from build123d import *

# Parameters (mm, degrees)
BOSS_EXTRUDE1_DEPTH     = 30
CUT_EXTRUDE1_DEPTH      = 72.944422994
CUT_EXTRUDE1_DEPTH_BACK = 4
SKETCH2_R               = 5
SKETCH3_R               = 2.25
CUT_EXTRUDE2_DEPTH      = 74.484692406
CHAMFER1_SIZE           = 1.5
SKETCH4_R               = 1.355
CUT_EXTRUDE3_DEPTH      = 10


with BuildPart() as part:
    # Sketch1 → Boss-Extrude1 (new body)
    with BuildSketch(Plane.XY):
        with BuildLine():
            Line((-35, -12), (-35, 12))
            ThreePointArc((-35, 12), (-34.414213562, 13.414213562), (-33, 14))
            Line((-33, 14), (33, 14))
            ThreePointArc((33, 14), (34.414213562, 13.414213562), (35, 12))
            Line((35, 12), (35, -12))
            ThreePointArc((35, -12), (35.585786438, -13.414213562), (37, -14))
            Line((37, -14), (45, -14))
            Line((45, -14), (45, 8))
            ThreePointArc((45, 8), (46.171572875, 10.828427125), (49, 12))
            Line((49, 12), (56, 12))
            ThreePointArc((56, 12), (58.828427125, 13.171572875), (60, 16))
            Line((60, 16), (60, 24))
            Line((60, 24), (33, 24))
            Line((33, 24), (-33, 24))
            Line((-33, 24), (-60, 24))
            Line((-60, 24), (-60, 16))
            ThreePointArc((-60, 16), (-58.828427125, 13.171572875), (-56, 12))
            Line((-56, 12), (-49, 12))
            ThreePointArc((-49, 12), (-46.171572875, 10.828427125), (-45, 8))
            Line((-45, 8), (-45, -14))
            Line((-45, -14), (-37, -14))
            ThreePointArc((-37, -14), (-35.585786438, -13.414213562), (-35, -12))
        make_face()
    extrude(amount=BOSS_EXTRUDE1_DEPTH)

    # Sketch2 → Cut-Extrude1 (cut, two sides: drawn at the far end of the back side and taken through both)
    with BuildSketch(Plane.XZ.offset(-12).offset(-CUT_EXTRUDE1_DEPTH_BACK)):
        with Locations(Location((-52.5, 15, 0), (0, 0, 134.427004004))):
            Circle(SKETCH2_R)
        with Locations(Location((52.5, 15, 0), (0, 0, 225.572995999))):
            Circle(SKETCH2_R)
    extrude(amount=CUT_EXTRUDE1_DEPTH + CUT_EXTRUDE1_DEPTH_BACK, mode=Mode.SUBTRACT)

    # Sketch3 → Cut-Extrude2 (cut, through all)
    with BuildSketch(Plane.XZ.offset(-16)):
        with Locations((-52.5, 15)):
            Circle(SKETCH3_R)
        with Locations((52.5, 15)):
            Circle(SKETCH3_R)
    extrude(amount=-CUT_EXTRUDE2_DEPTH, mode=Mode.SUBTRACT)

    # Chamfer1
    chamfer1_edges = [part.edges().sort_by_distance(p)[0] for p in [
        (-54.75, 16, 15),
        (50.25, 16, 15),
    ]]
    chamfer(chamfer1_edges, length=CHAMFER1_SIZE)

    # Sketch4 → Cut-Extrude3 (cut)
    with BuildSketch(Plane.XZ.offset(14)):
        with Locations(Location((-40, 15, 0), (0, 0, 270))):
            Circle(SKETCH4_R)
        with Locations(Location((40, 15, 0), (0, 0, 270))):
            Circle(SKETCH4_R)
    extrude(amount=-CUT_EXTRUDE3_DEPTH, mode=Mode.SUBTRACT)


solid = part.part
Geometry check sheet. Reference: the model listing, model coordinates, mm. A direction names the side the tool comes from. Round coordinates to 2 decimals unless told otherwise and drop trailing zeros. Loops run counter-clockwise (first coordinate to the right, second up) from the corner with the lowest first, then second, coordinate; pieces in that order, holes last.
Item 1: Cross-section at C-C on z = 27. Record the boundary of the cut face in (x, y), then the cut area to 3 significant figures.
Item 2: Cross-section at A-A on x = 52.5. Record the boundary of the cut face in (y, z).
Item 3: Gauge pin test, flat ends, axial feed: pin 1 (0.8 mm diameter, centred on x = 39.5, z = 14.5, fed in from -Y); pin 2 (8 mm diameter, centred on y = 12.5, z = 13, fed in from +X); pin 3 (2 mm diameter, centred on x = -52.5, z = 8, fed in from -Y); pin 4 (3.5 mm diameter, centred on x = 52.5, z = 15, fed in from +Y). Record the tip position at first contact, or that the pin passes through.
Item 4: Cross-section at D-D on x = -40. Record the boundary of the cut face in (y, z) (3 decimals), then the cut area to 3 significant figures.
Item 5: Thickness scan on line 1 (X direction, y = -11, z = 15) (3 decimals); line 2 (Z direction, x = -52, y = 13); line 3 (X direction, y = -8, z = 2.5). Record the ranges inside material, lowest first.
Item 6: Access from +Z, -Z, +X, -X, +Y, -Y to the whole of each face (thin tool, end or side, straight path). Record for faces 1 (the flat face through (0, 14, 15)), 2 (the cylindrical face through (47.717, 13.884, 16.457)), 3 (the flat face through (52, 12, 24)), 4 (the flat face through (-42, -14, 15)), 5 (the flat face through (-53, 12, 24)).
Item 7: Mould release check, pull along Z, two halves, no side actions. Record for faces 6 (the cylindrical face through (-54.748, 20.704, 15.099)), 7 (the flat face through (-1, 18, 30)), 8 (the cylindrical face through (-46.203, 10.859, 14.79)): pulls with the +Z half, pulls with the -Z half, needs draft (parallel to the pull), parting line crosses it, or undercut.
Item 8: Cross-section at B-B on y = 0. Record the boundary of the cut face in (x, z), then the cut area to 3 significant figures.
Answer sheet:
1. outline: (-60, 16) arc R4 ccw to (-56, 12) - (-49, 12) arc R4 cw to (-45, 8) - (-45, -14) - (-37, -14) arc R2 ccw to (-35, -12) - (-35, 12) arc R2 cw to (-33, 14) - (33, 14) arc R2 cw to (35, 12) - (35, -12) arc R2 ccw to (37, -14) - (45, -14) - (45, 8) arc R4 cw to (49, 12) - (56, 12) arc R4 ccw to (60, 16) - (60, 24) - (-60, 24) - close
1. area: 1,820 mm2
2. outline: (12, 0) - (24, 0) - (24, 12.75) - (17.5, 12.75) - (16, 11.25) - (16, 10) - (12, 10) - close; (12, 20) - (16, 20) - (16, 18.75) - (17.5, 17.25) - (24, 17.25) - (24, 30) - (12, 30) - close
3. pin 1: stops at y = -4
3. pin 2: stops at x = 60
3. pin 3: stops at y = 12
3. pin 4: passes through
4. outline: (-14, 0) - (24, 0) - (24, 30) - (-14, 30) - (-14, 16.355) - (-4, 16.355) - (-4, 13.645) - (-14, 13.645) - close
4. area: 1,110 mm2
5. line 1: x = -45 to -41.355, -38.645 to -35, 35 to 38.645, 41.355 to 45
5. line 2: z = 0 to 10.03, 19.97 to 30
5. line 3: x = -45 to -35, 35 to 45
6. face 1: +Z, -Z, -Y
6. face 2: -Y
6. face 3: +Z, -Z, +X, -Y
6. face 4: +Z, -Z, +X, -X, -Y
6. face 5: +Z, -Z, -X, -Y
7. face 6: undercut
7. face 7: pulls with the +Z half
7. face 8: needs draft
8. outline: (-45, 0) - (-35, 0) - (-35, 30) - (-45, 30) - close; (35, 0) - (45, 0) - (45, 30) - (35, 30) - close
8. area: 600 mm2
